Part model, mm, in its own coordinate system. Round coordinates to 2 decimals unless told otherwise and drop trailing zeros. Order: outer loops, then holes, each group sorted by start corner. A loop starts at its lowest first (then second) coordinate and runs counter-clockwise, first axis right, second up. Notation, with made-up numbers: (56, -10.5) -> (104, -10.5) arc R32 cw to (104, 24.5) -> close; hole circle Ø11 at (-37, 20.25). An arc over 180 degrees is marked (long way). Use CSV: the item, a comma, the result in double quotes.
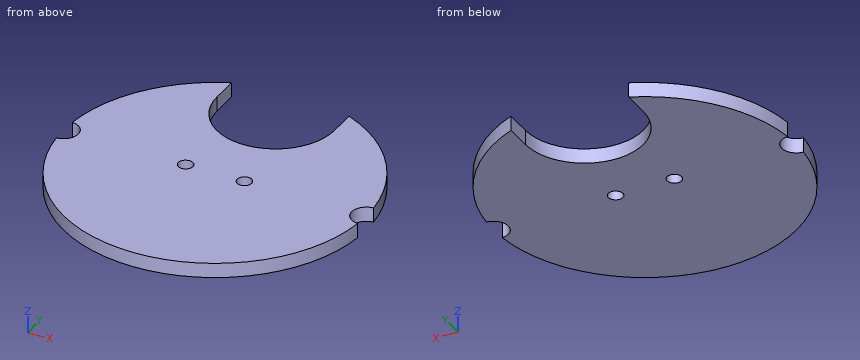
```python
from build123d import *

# Parameters (mm, degrees)
SKETCH1_R      = 65.405
EXTRUDE1_DEPTH = 6.35
SKETCH2_R      = 6.35
SKETCH2_R_2    = 3.175
EXTRUDE2_DEPTH = 93.714349213


with BuildPart() as part:
    # Sketch1 → Extrude1 (new body)
    with BuildSketch(Plane.XY):
        Circle(SKETCH1_R)
    extrude(amount=EXTRUDE1_DEPTH)

    # Sketch2 → Extrude2 (cut, through all)
    with BuildSketch(Plane.XY.offset(6.35)):
        with Locations((-65.405, 0)):
            Circle(SKETCH2_R)
        with Locations((65.405, 0)):
            Circle(SKETCH2_R)
        with Locations((12.7, 0)):
            Circle(SKETCH2_R_2)
        with Locations((-12.7, 0)):
            Circle(SKETCH2_R_2)
        with BuildLine():
            Line((-25.4, 48.509773864), (-25.4, 60.271502595))
            Line((-25.4, 60.271502595), (-25.4, 72.027407772))
            Line((-25.4, 72.027407772), (25.4, 72.027407772))
            Line((25.4, 72.027407772), (25.4, 60.271502595))
            Line((25.4, 60.271502595), (25.4, 48.509773864))
            ThreePointArc((25.4, 48.509773864), (0, 23.109773864), (-25.4, 48.509773864))
        make_face()
    extrude(amount=-EXTRUDE2_DEPTH, mode=Mode.SUBTRACT)


solid = part.part
```
(1) Cut at C-C, the plane y = -42. Give the cut face in (x, z), then the cut area to 3 significant figures.
Reply:
outline,"(-50.14, 0) -> (50.14, 0) -> (50.14, 6.35) -> (-50.14, 6.35) -> close"
area,"637 mm2"
(2) Drop flat-ended pins along their axis: P1, Ø2, axis at x = -2.5, z = 5.5, coming from the +Y side; P2, Ø1.5, axis at y = 15, z = 2.5, coming from the +X side; P3, Ø1.5, axis at x = 42.5, z = 3, coming from the +Y side. Give the stop position or say it passes through.
Reply:
P1,"y = 23.35"
P2,"x = 63.83"
P3,"y = 50.35"
(3) Probe probe 1 along X at (y, z) = (2.5, 4); probe 2 along Y at (x, z) = (-12.7, 3.75) (3 decimals); probe 3 along X at (y, z) = (0.5, 3.5). List the from-to ranges inside material, lowest first. Write a range as [from, to].
Reply:
probe 1,"[-59.57, -14.66], [-10.74, 10.74], [14.66, 59.57]"
probe 2,"[-64.16, -3.175], [3.175, 26.513]"
probe 3,"[-59.07, -15.84], [-9.56, 9.56], [15.84, 59.07]"
(4) Cut at B-B, the plane x = -12.7. Give the cut face in (y, z) (3 decimals).
Reply:
outline,"(-64.16, 0) -> (-3.175, 0) -> (-3.175, 6.35) -> (-64.16, 6.35) -> close; (3.175, 0) -> (26.513, 0) -> (26.513, 6.35) -> (3.175, 6.35) -> close"
(5) Cut at A-A, the plane z = 2.75. State how many separate pieces and enclosed holes the cut face has, then the cut area to 3 significant figures.
Reply:
separate pieces,"1"
enclosed holes,"2"
area,"11,500 mm2"
(6) Cut at D-D, the plane x = 35. Give the cut face in (y, z), then the cut area to 3 significant figures.
Reply:
outline,"(-55.25, 0) -> (55.25, 0) -> (55.25, 6.35) -> (-55.25, 6.35) -> close"
area,"702 mm2"
